```python
from build123d import *

# Parameters (mm, degrees)
F1_DEPTH = 25.4
F2_W     = 57.15
F2_H     = 25.4
F3_DEPTH = 76.2
F4_W     = 57.15
F4_H     = 25.4
F5_DEPTH = 114.3
F6_W     = 57.15
F6_H     = 25.4
F7_DEPTH = 114.3
F8_W     = 228.6
F8_H     = 25.4
F9_DEPTH = 279.4


with BuildPart() as f1:
    # F0 (on Front) → F1 (new body)
    with BuildSketch(Plane.XZ):
        Polygon((-171.4900614394, 291.4170305759), (-228.6400614394, 291.4170305759), (-228.6400614394, -318.1829694241), (-0.0400614394, -318.1829694241), (-0.0400614394, 291.4170305759), (-57.1900614394, 291.4170305759), (-57.1900614394, 139.0170305759), (-171.4900614394, 139.0170305759), align=None)
    extrude(amount=F1_DEPTH)

    # F2 (on face) → F3 (join)
    with BuildSketch(Plane(origin=(0, 0, 0), x_dir=(-1, 0, 0), z_dir=(0, 1, 0))):
        with Locations((28.6150614394, 278.7170305759)):
            Rectangle(F2_W, F2_H)
        with Locations((200.0650614394, 278.7170305759)):
            Rectangle(F2_W, F2_H)
    extrude(amount=F3_DEPTH)

    # F4 (on face) → F5 (join)
    with BuildSketch(Plane.XY.offset(291.4170305759)):
        with Locations((-28.6150614394, 88.9)):
            Rectangle(F4_W, F4_H)
    extrude(amount=-F5_DEPTH)

    # F6 (on face) → F7 (join)
    with BuildSketch(Plane.XY.offset(291.4170305759)):
        with Locations((-200.0650614394, 88.9)):
            Rectangle(F6_W, F6_H)
    extrude(amount=-F7_DEPTH)

    # F8 (on face) → F9 (join)
    with BuildSketch(Plane.XZ.offset(25.4)):
        with Locations((-114.3400614394, -102.2829694241)):
            Rectangle(F8_W, F8_H)
    extrude(amount=F9_DEPTH)


solid = f1.part
```
The listing builds one solid part. Answer for the finished solid, in the listing's coordinates (mm). A direction names the side the tool comes from. Give positions to 0.01 mm unless a question says otherwise; leave off trailing zeros. Order: outer loops, then holes, each group sorted by start corner. A loop starts at its lowest first (then second) coordinate and runs counter-clockwise, first axis right, second up.
1) Find section A-A on z = 185. Write down the section's boundary in (x, y), then the cut area to 3 significant figures.
Reported:
outline: (-228.64, -25.4) - (-171.49, -25.4) - (-171.49, 0) - (-228.64, 0) - close; (-228.64, 76.2) - (-171.49, 76.2) - (-171.49, 101.6) - (-228.64, 101.6) - close; (-57.19, -25.4) - (-0.04, -25.4) - (-0.04, 0) - (-57.19, 0) - close; (-57.19, 76.2) - (-0.04, 76.2) - (-0.04, 101.6) - (-57.19, 101.6) - close
area: 5,810 mm2
2) For faces 5 (the face through (-29, 89, 177.117)), 6 (the face through (-116, -25.4, -215)), 7 (the face through (-114, -13, 139.017)), 8 (the face through (-116, -25.4, 61)), 9 (the face through (-200, 38, 266.017)), determine the directions among +Z, -Z, +X, -X, +Y, -Y from which every point of the face is accessible in a straight line to the end or side of a thin tool.
Reported:
face 5: -Z, +X, -X, +Y
face 6: -Z, +X, -X, -Y
face 7: +Z, +Y, -Y
face 8: +Z, +X, -X, -Y
face 9: -Z, +X, -X
3) Find section D-D on z = 5. Write down the section's boundary in (x, y), then the cut area to 3 significant figures.
Reported:
outline: (-228.64, -25.4) - (-0.04, -25.4) - (-0.04, 0) - (-228.64, 0) - close
area: 5,810 mm2
4) Given P1, Ø20.5, axis at x = -196, y = 87.5, coming from the -Z side; P2, Ø2, axis at x = -121.5, z = 138, coming from the -Y side; P3, Ø4, axis at x = -48, y = -201, coming from the +Z side, each flat-ended and moving along its own axis, determine where each tip first touches the part or whether it passes through.
Reported:
P1: stops at z = 177.12
P2: stops at y = -25.4
P3: stops at z = -89.58
5) Consider line 1 along Y through (x, z) = (-44, 239); line 2 along Y through (x, z) = (-155, 64); line 3 along Z through (x, y) = (-92.5, -44). Determine where each line is inside the solid, lowest interval first.
Reported:
line 1: y = -25.4 to 0, 76.2 to 101.6
line 2: y = -25.4 to 0
line 3: z = -114.98 to -89.58
6) Find section C-C on y = -18. Write down the section's boundary in (x, z).
Reported:
outline: (-228.64, -318.18) - (-0.04, -318.18) - (-0.04, 291.42) - (-57.19, 291.42) - (-57.19, 139.02) - (-171.49, 139.02) - (-171.49, 291.42) - (-228.64, 291.42) - close
7) Determine the mould class of faces 1 (the face through (-171.49, 37, 267)), 2 (the face through (-228.64, -12, 33)), 3 (the face through (-0.04, -12, 33)), 4 (the face through (-116, 0, -22)) for opening direction X: pulls with the +X half, pulls with the -X half, needs draft (parallel to the pull), parting line crosses it, or undercut.
Reported:
face 1: undercut
face 2: pulls with the -X half
face 3: pulls with the +X half
face 4: needs draft
8) Find section B-B on x = -40. Write down the section's boundary in (y, z), then the cut area to 3 significant figures.
Reported:
outline: (-304.8, -114.98) - (-25.4, -114.98) - (-25.4, -318.18) - (0, -318.18) - (0, 266.02) - (76.2, 266.02) - (76.2, 177.12) - (101.6, 177.12) - (101.6, 291.42) - (-25.4, 291.42) - (-25.4, -89.58) - (-304.8, -89.58) - close
area: 27,400 mm2
